Build history of the part. All positions in model axes, mm. A direction names the side the tool comes from. Give positions to 0.01 mm unless a question says otherwise; leave off trailing zeros. Order: outer loops, then holes, each group sorted by start corner. A loop starts at its lowest first (then second) coordinate and runs counter-clockwise, first axis right, second up. Notation, with made-up numbers: (62.5, 4.5) -> (81.5, 4.5) arc R22 cw to (81.5, 14.5) -> close; hole circle Ø3 at (-3.5, -2). An arc over 180 degrees is marked (long way). One line per question, with ' | ' between items. Start each with the question number.
(1) Cut at B-B (y = 0.85). Give the cut face in (x, z), then the cut area to 3 significant figures.
(2) Pin check, flat tip, straight feed: pin 1 Ø2 at (x, z) = (6.5, 0) entering from +Y. Stop position of the tip, or through.
(3) Pull direction X, two halves, no side cores. Call faces 4 (the face through (0, 1.27, -1)), 5 (the face through (5.08, 1, 2)), 6 (the face through (-10.16, 1, -1)): +X half, -X half, draft (parallel to the pull), parting line (faces both ways), or undercut.
(4) Drill centre lines: L1, parallel to X at y = 0.2, z = 0.25; L2, parallel to Z at x = 0.75, y = 1.75; L3, parallel to Y at x = 0, z = -3.5. Where is each one in solid material? Low to high. Write a range as from..to.
(5) Cut at C-C (x = 6.5). Give the cut face in (y, z), then the cut area to 3 significant figures.
(6) Which spindle directions (+Z, -Z, +X, -X, +Y, -Y) get a long thin tool onto all of the face, cutting with end or side? Do faces 1 (the face through (0, 2, -4.286)), 2 (the face through (-8, 1, 3.81)), 3 (the face through (-5.08, 1, 2)). Say none if no direction does.
(7) Cut at A-A (z = 0.25). Give the cut face in (x, y).
(8) Cut at D-D (z = -1). Give the cut face in (x, y), then the cut area to 3 significant figures.
from build123d import *

# Parameters (mm, degrees)
SKETCH1_W           = 20.32
SKETCH1_H           = 10.16
BOSS_EXTRUDE1_DEPTH = 1.27
SKETCH2_W           = 10.16
SKETCH2_H           = 5.08
CUT_EXTRUDE1_DEPTH  = 12.43
SKETCH4_W           = 20.32
SKETCH4_H           = 0.79375
BOSS_EXTRUDE2_DEPTH = 1.27
SKETCH5_W           = 5.08
SKETCH5_H           = 1.27
CUT_EXTRUDE2_DEPTH  = 1.27


with BuildPart() as part:
    # Sketch1 → Boss-Extrude1 (new body)
    with BuildSketch(Plane(origin=(0, 0, 0), x_dir=(1, 0, 0), z_dir=(0, 1, 0))):
        Rectangle(SKETCH1_W, SKETCH1_H)
    extrude(amount=BOSS_EXTRUDE1_DEPTH)

    # Sketch2 → Cut-Extrude1 (cut, through all)
    with BuildSketch(Plane(origin=(0, 1.27, 0), x_dir=(1, 0, 0), z_dir=(0, 1, 0))):
        with Locations((0, -2.54)):
            Rectangle(SKETCH2_W, SKETCH2_H)
    extrude(amount=-CUT_EXTRUDE1_DEPTH, mode=Mode.SUBTRACT)

    # Sketch4 → Boss-Extrude2 (add)
    with BuildSketch(Plane(origin=(0, 1.27, 0), x_dir=(1, 0, 0), z_dir=(0, 1, 0))):
        with Locations((0, 4.683125)):
            Rectangle(SKETCH4_W, SKETCH4_H)
    extrude(amount=BOSS_EXTRUDE2_DEPTH)

    # Sketch5 → Cut-Extrude2 (cut)
    with BuildSketch(Plane.XY.offset(5.08)):
        with Locations((7.62, 0.635)):
            Rectangle(SKETCH5_W, SKETCH5_H)
        with Locations((-7.62, 0.635)):
            Rectangle(SKETCH5_W, SKETCH5_H)
    extrude(amount=-CUT_EXTRUDE2_DEPTH, mode=Mode.SUBTRACT)


solid = part.part
Result set:
1) outline: (-10.16, -5.08) -> (10.16, -5.08) -> (10.16, 3.81) -> (5.08, 3.81) -> (5.08, 0) -> (-5.08, 0) -> (-5.08, 3.81) -> (-10.16, 3.81) -> close | area: 142 mm2
2) pin 1: stops at y = 1.27
3) face 4: draft | face 5: undercut | face 6: -X half
4) L1: x = -10.16..-5.08, 5.08..10.16 | L2: z = -5.08..-4.29 | L3: y = 0..1.27
5) outline: (0, -5.08) -> (2.54, -5.08) -> (2.54, -4.29) -> (1.27, -4.29) -> (1.27, 3.81) -> (0, 3.81) -> close | area: 12.3 mm2
6) face 1: +Z, +X, -X, +Y | face 2: +Z, +X, -X, +Y, -Y | face 3: +Z, +Y, -Y
7) outline: (-10.16, 0) -> (-5.08, 0) -> (-5.08, 1.27) -> (-10.16, 1.27) -> close; (5.08, 0) -> (10.16, 0) -> (10.16, 1.27) -> (5.08, 1.27) -> close
8) outline: (-10.16, 0) -> (10.16, 0) -> (10.16, 1.27) -> (-10.16, 1.27) -> close | area: 25.8 mm2
